Autodesk Inventor part; units mm, degrees
ref_plane "YZ Plane" through (0, 0, 0) normal (1, 0, 0) x (0, 1, 0)
ref_plane "XZ Plane" through (0, 0, 0) normal (0, 1, 0) x (-1, 0, 0)
ref_plane "XY Plane" through (0, 0, 0) normal (0, 0, 1) x (1, 0, 0)
sketch "Sketch1" plane through (0, 0, 0) normal (0, 0, 1) x (1, 0, 0)
  line L0 (-83, 53) -> (83, 53) construction
  line L1 (83, 53) -> (83, -53) construction
  line L2 (83, -53) -> (-83, -53) construction
  line L3 (-83, -53) -> (-83, 53) construction
  line L4 (-83, 53) -> (83, -53) construction
  line L5 (83, 53) -> (-83, -53) construction
  line L6 (-91, 61) -> (91, 61)
  line L7 (91, 61) -> (91, -61)
  line L8 (91, -61) -> (-91, -61)
  line L9 (-91, -61) -> (-91, 61)
  line L10 (-91, 61) -> (91, -61) construction
  line L11 (-91, -61) -> (91, 61) construction
  point P0 (0, 0)
  point P1 (0, 0)
  point P2 (0, 0)
  dimension "d0" = 166
  dimension "d1" = 106
  dimension "d2" = 8
  dimension "d3" = 8
extrude "Extrusion1" add sketch "Sketch1" along normal blind 3
sketch "Sketch2" plane through (0, 0, 3) normal (0, 0, 1) x (1, 0, 0)
  line L0 (-83, 53) -> (83, 53)
  line L1 (83, 53) -> (83, -53)
  line L2 (83, -53) -> (-83, -53)
  line L3 (-83, -53) -> (-83, 53)
  line L4 (-83, 53) -> (83, -53) construction
  line L5 (83, 53) -> (-83, -53) construction
  line L6 (-80, 50) -> (80, 50)
  line L7 (80, 50) -> (80, -50)
  line L8 (80, -50) -> (-80, -50)
  line L9 (-80, -50) -> (-80, 50)
  line L10 (-80, -50) -> (80, 50) construction
  line L11 (80, -50) -> (-80, 50) construction
  point P0 (0, 0)
  point P1 (0, 0)
  point P2 (0, 0)
  dimension "d6" = 166
  dimension "d7" = 106
  dimension "d8" = 3
  dimension "d9" = 3
extrude "Extrusion2" add sketch "Sketch2" along normal blind 3
fillet "Fillet1" radius 3 4 edges at (80, 50, 4.5) (80, -50, 4.5) (-80, -50, 4.5) (-80, 50, 4.5)
fillet "Fillet2" radius 6 4 edges at (83, 53, 4.5) (83, -53, 4.5) (-83, -53, 4.5) (-83, 53, 4.5)
sketch "Sketch3" plane through (0, 0, 0) normal (0, 0, -1) x (-1, 0, 0)
  line L0 (91, 61) -> (-91, 61)
  line L1 (-91, 61) -> (-91, -61)
  line L2 (91, -61) -> (91, 61)
  circle A0 centre (-85, 55) radius 2
  line L3 (0, 0) -> (-15.5328, 0) construction
  line L4 (0, 0) -> (0, 8.2904) construction
  circle A1 centre (-85, -55) radius 2
  circle A2 centre (85, 55) radius 2
  circle A3 centre (85, -55) radius 2
  dimension "d14" = 4
  dimension "d15" = 6
  dimension "d16" = 6
hole "Hole1" at (85, 55, 0) at (85, -55, 0) at (-85, -55, 0) at (-85, 55, 0) direction (0, 0, 1) diameter 4.5 depth 8 tip angle 118
sketch "Sketch4" plane through (0, 0, 3) normal (0, 0, 1) x (1, 0, 0)
  line L0 (-80, 47) -> (-80, -47)
  line L1 (-77, -50) -> (77, -50)
  line L2 (77, 50) -> (-77, 50)
  line L3 (0, 0) -> (-11.513, 0) construction
  line L4 (0, 0) -> (0, -7.6384) construction
  circle A0 centre (-72, -42) radius 5.1497
  circle A1 centre (-72, 42) radius 5.1497
  circle A2 centre (72, -42) radius 5.1497
  circle A3 centre (72, 42) radius 5.1497
  dimension "d24" = 8
  dimension "d25" = 8
hole "Hole2" at (-72, -42, 3) at (-72, 42, 3) at (72, -42, 3) at (72, 42, 3) direction (0, 0, -1) diameter 4.5 depth 8 tip angle 118
sketch "Sketch5" plane through (0, 0, 3) normal (0, 0, 1) x (1, 0, 0)
  circle A0 centre (72, 42) radius 2.25
  circle A1 centre (72, -42) radius 2.25
  circle A2 centre (-72, 42) radius 2.25
  circle A3 centre (-72, -42) radius 2.25
  arc A4 (-77, 50) -> (-80, 47) centre (-77, 47) ccw
  line L0 (-80, 47) -> (-80, -47)
  arc A5 (-80, -47) -> (-77, -50) centre (-77, -47) ccw
  line L1 (-77, -50) -> (77, -50)
  arc A6 (77, -50) -> (80, -47) centre (77, -47) ccw
  line L2 (80, -47) -> (80, 47)
  arc A7 (80, 47) -> (77, 50) centre (77, 47) ccw
  line L3 (77, 50) -> (-77, 50)
  circle A8 centre (-25, -40) radius 0.5
  circle A9 centre (-40, -15) radius 0.5
  circle A10 centre (-45, 5) radius 0.5
  circle A11 centre (-45, 20) radius 0.5
  circle A12 centre (35, -40) radius 0.5
  circle A13 centre (25, 25) radius 0.5
  circle A14 centre (25, 40) radius 0.5
  point P0 (0, 0)
  dimension "d33" = 1
  dimension "d34" = 1
  dimension "d35" = 1
  dimension "d36" = 1
  dimension "d37" = 1
  dimension "d38" = 1
  dimension "d39" = 1
  dimension "d41" = 55
  dimension "d43" = 40
  dimension "d44" = 35
  dimension "d45" = 35
  dimension "d50" = 55
  dimension "d51" = 55
  dimension "d53" = 45
  dimension "d54" = 30
  dimension "d55" = 45
  dimension "d56" = 35
  dimension "d57" = 10
  dimension "d58" = 10
  dimension "d59" = 25
  dimension "d60" = 10
equation "\"d15\" = 1.5 * d14"
equation "\"d16\" = 1.5 * d14"
properties part number "Base.Box.Lid"
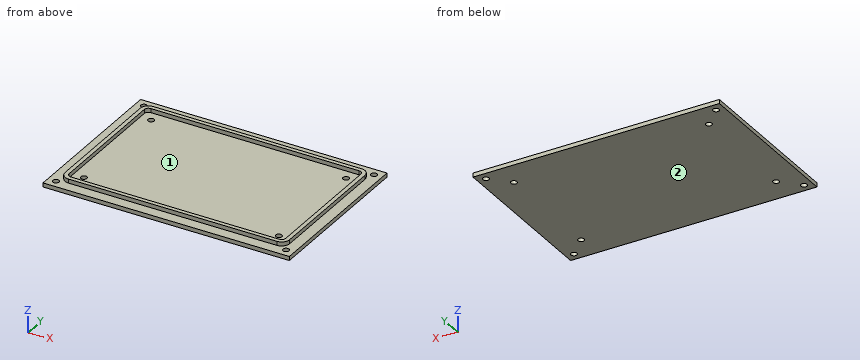
Check sheet for the modelled part. Datum: model origin and axes. Units: mm. Face numbers are marked on the shaded views. A direction names the side the tool comes from. Give positions to 0.01 mm unless a question says otherwise; leave off trailing zeros. Loops run counter-clockwise (first coordinate to the right, second up) from the corner with the lowest first, then second, coordinate; pieces in that order, holes last. Notation, with made-up numbers: M 32.25,56 L 87.25,56 A19 cw 87.25,91 Z; hole C -14.5,74.5 d11. An arc over 180 degrees is marked long. Answer as a JSON object with one key per item and string values. Group by question number.
Q1. Material ranges on line 1 along X through (y, z) = (-42, 1.05); line 2 along Y through (x, z) = (85, 2); line 3 along Y through (x, z) = (72, 2.05), recorded low to high. Write a range as [from, to].
Q2. Access from +Z, -Z, +X, -X, +Y, -Y to the whole of each face (thin tool, end or side, straight path). Record for the marked faces 1 and 2.
Q3. Cross-section at C-C on z = 4.25. Record the cut outline in (x, y).
Q4. Cross-section at B-B on y = 55. Record the cut outline in (x, z), then the cut area to 3 significant figures.
Q5. Cross-section at A-A on x = -72. Record the cut outline in (y, z), then the cut area to 3 significant figures.
Q6. Go/stop test with flat-tipped pins: P1, Ø2.5, axis at x = 85, y = -55, coming from the +Z side; P2, Ø1.5, axis at x = -34.5, y = -34.5, coming from the +Z side; P3, Ø10, axis at x = 71, y = 11.5, coming from the -Z side; P4, Ø1.5, axis at x = 25.5, z = 4.5, coming from the +Y side. Record where each tip stops, or that it passes through.
Q7. Cross-section at D-D on y = -29.5. Record the cut outline in (x, z), then the cut area to 3 significant figures.
Evaluation:
{
 "1": {"line 1": "x = [-91, -74.25], [-69.75, 69.75], [74.25, 91]", "line 2": "y = [-61, -57.25], [-52.75, 52.75], [57.25, 61]", "line 3": "y = [-61, -44.25], [-39.75, 39.75], [44.25, 61]"},
 "2": {"face 1": "+Z", "face 2": "-Z, +X, -X, +Y, -Y"},
 "3": {"outline": "M -83,-47 A6 ccw -77,-53 L 77,-53 A6 ccw 83,-47 L 83,47 A6 ccw 77,53 L -77,53 A6 ccw -83,47 Z; hole M -80,-47 A3 ccw -77,-50 L 77,-50 A3 ccw 80,-47 L 80,47 A3 ccw 77,50 L -77,50 A3 ccw -80,47 Z"},
 "4": {"outline": "M -91,0 L -87.25,0 L -87.25,3 L -91,3 Z; M -82.75,0 L 82.75,0 L 82.75,3 L -82.75,3 Z; M 87.25,0 L 91,0 L 91,3 L 87.25,3 Z", "area": "519 mm2"},
 "5": {"outline": "M -61,0 L -44.25,0 L -44.25,3 L -50,3 L -50,6 L -53,6 L -53,3 L -61,3 Z; M -39.75,0 L 39.75,0 L 39.75,3 L -39.75,3 Z; M 44.25,0 L 61,0 L 61,3 L 53,3 L 53,6 L 50,6 L 50,3 L 44.25,3 Z", "area": "357 mm2"},
 "6": {"P1": "passes through", "P2": "stops at z = 3", "P3": "stops at z = 0", "P4": "stops at y = 53"},
 "7": {"outline": "M -91,0 L 91,0 L 91,3 L 83,3 L 83,6 L 80,6 L 80,3 L -80,3 L -80,6 L -83,6 L -83,3 L -91,3 Z", "area": "564 mm2"}
}
